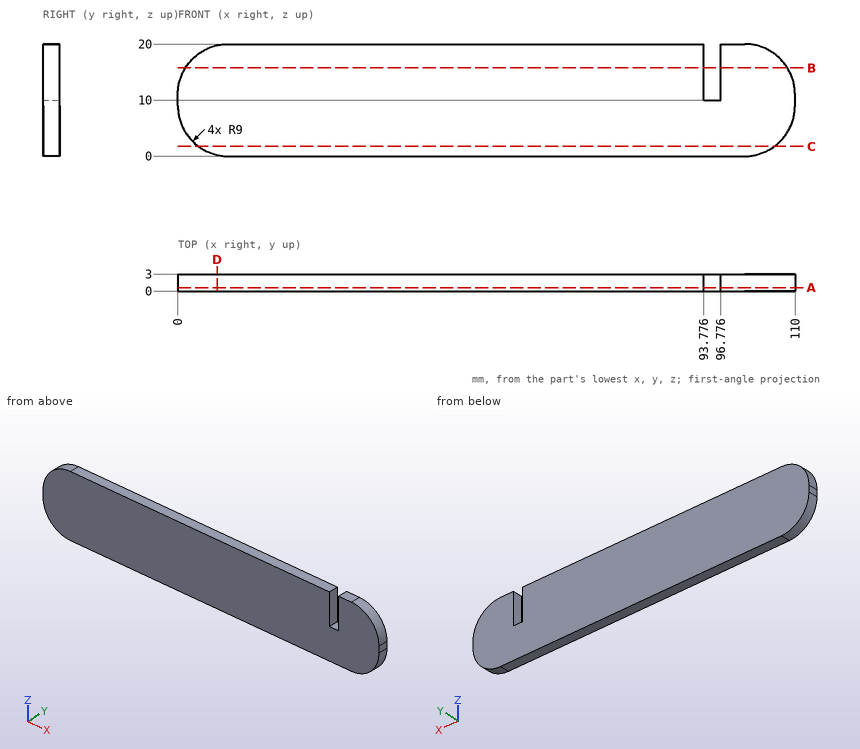
Geometry: see drawing. Coordinates: mm, zero at the bounding-box minimum. Coordinates: 2 decimals unless noted, no trailing zeros. Loops run counter-clockwise (first coordinate to the right, second up) from the corner with the lowest first, then second, coordinate; pieces in that order, holes last. Notation, with made-up numbers: M 80.5,63 L 103.5,63 A18 ccw 103.5,93 Z; hole C -2,86.25 d6. An arc over 180 degrees is marked long. Put each result on its own line as item: value. Start each with the question number.
1) Cut plane C-C on z = 1.75. Return the cut outline in (x, y), then the cut area to 3 significant figures.
2) Cut plane A-A on y = 0.6. Return the cut outline in (x, z).
3) Cut plane B-B on z = 15.75. Return the cut outline in (x, y) (1 decimal).
4) Ray query, L1, parallel to X at y = 1.5, z = 15.5 (1 decimal); L2, parallel to X at y = 2.85, z = 14.5 (1 decimal); L3, parallel to X at y = 1.05, z = 5.5. Return the intervals inside material, ascending. Write a range as from..to.
5) Cut plane D-D on x = 7. Return the cut outline in (y, z) (1 decimal).
The answers:
1. outline: M 3.67,0 L 106.33,0 L 106.33,3 L 3.67,3 Z
1. area: 308 mm²
2. outline: M 0,9 A9 ccw 9,0 L 101,0 A9 ccw 110,9 L 110,11 A9 ccw 101,20 L 96.78,20 L 96.78,10 L 93.78,10 L 93.78,20 L 9,20 A9 ccw 0,11 Z
3. outline: M 1.4,0 L 93.8,0 L 93.8,3 L 1.4,3 Z; M 96.8,0 L 108.6,0 L 108.6,3 L 96.8,3 Z
4. L1: x = 1.2..93.8, 96.8..108.8
4. L2: x = 0.7..93.8, 96.8..109.3
4. L3: x = 0.71..109.29
5. outline: M 0,0.2 L 3,0.2 L 3,19.8 L 0,19.8 Z
